Build history of the part. All positions in model axes, mm. Face numbers are marked on the shaded views. Coordinates: 2 decimals unless noted, no trailing zeros. Write each loop counter-clockwise with the first axis right and the second up, starting at its lowest first coordinate (ties: lowest second). Pieces come first, ordered by that corner, then holes.
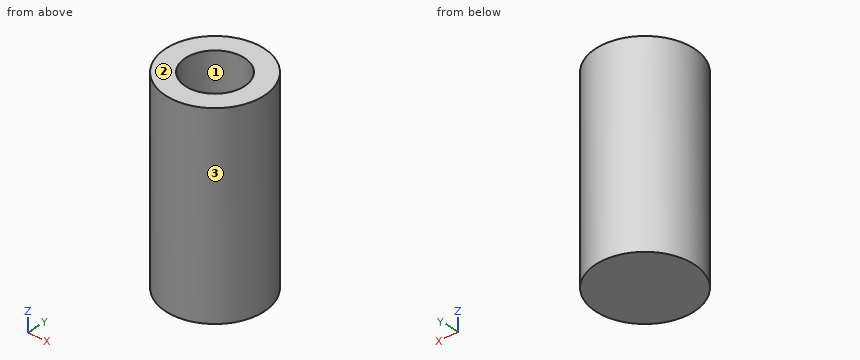
from build123d import *

# Parameters (mm, degrees)
F0_R     = 5
F1_DEPTH = 20
F2_R     = 3
F3_DEPTH = 10
F4_DEPTH = 10


with BuildPart() as f1:
    # F0 (on Top) → F1 (new body)
    with BuildSketch(Plane.XY):
        Circle(F0_R)
    extrude(amount=F1_DEPTH)

    # F2 (on face) → F3 (cut)
    with BuildSketch(Plane.XY.offset(20)):
        Circle(F2_R)
    extrude(amount=F3_DEPTH, mode=Mode.SUBTRACT)

    # F2 (on face) → F4 (cut)
    with BuildSketch(Plane.XY.offset(20)):
        Circle(F2_R)
    extrude(amount=-F4_DEPTH, mode=Mode.SUBTRACT)


solid = f1.part
(1) Slice it at C-C, the plane z = 12. List the corners of the cut face in (x, y).
(2) Probe L1, parallel to Y at x = 0, z = 14.5; L2, parallel to Z at x = -0.75, y = -1; L3, parallel to X at y = 1.25, z = 16. List the from-to ranges inside material, lowest first.
(3) Slice it at A-A, the plane x = 0. List the corners of the cut face in (y, z), and give its area (3 significant figures).
(4) Slice it at D-D, the plane z = 5.5. List the corners of the cut face in (x, y), and give its area (3 significant figures).
(5) Two-plate mould, pull along Y, no slides. Class the marked faces 1, 2 and 3: pulls with the +Y half, pulls with the -Y half, needs draft (parallel to the pull), parting line crosses it, or undercut.
(6) Flat gauge pin, fed straight in: P1, Ø2, axis at x = 4, y = 4, coming from the -Z side. Where does the tip first touch, or does it go through?
Results:
1. outline: circle Ø10 at (0, 0); hole circle Ø6 at (0, 0)
2. L1: y = -5 to -3, 3 to 5
2. L2: z = 0 to 10
2. L3: x = -4.84 to -2.73, 2.73 to 4.84
3. outline: (-5, 0) - (5, 0) - (5, 20) - (3, 20) - (3, 10) - (-3, 10) - (-3, 20) - (-5, 20) - close
3. area: 140 mm2
4. outline: circle Ø10 at (0, 0)
4. area: 78.5 mm2
5. face 1: undercut
5. face 2: needs draft
5. face 3: parting line crosses it
6. P1: stops at z = 0
